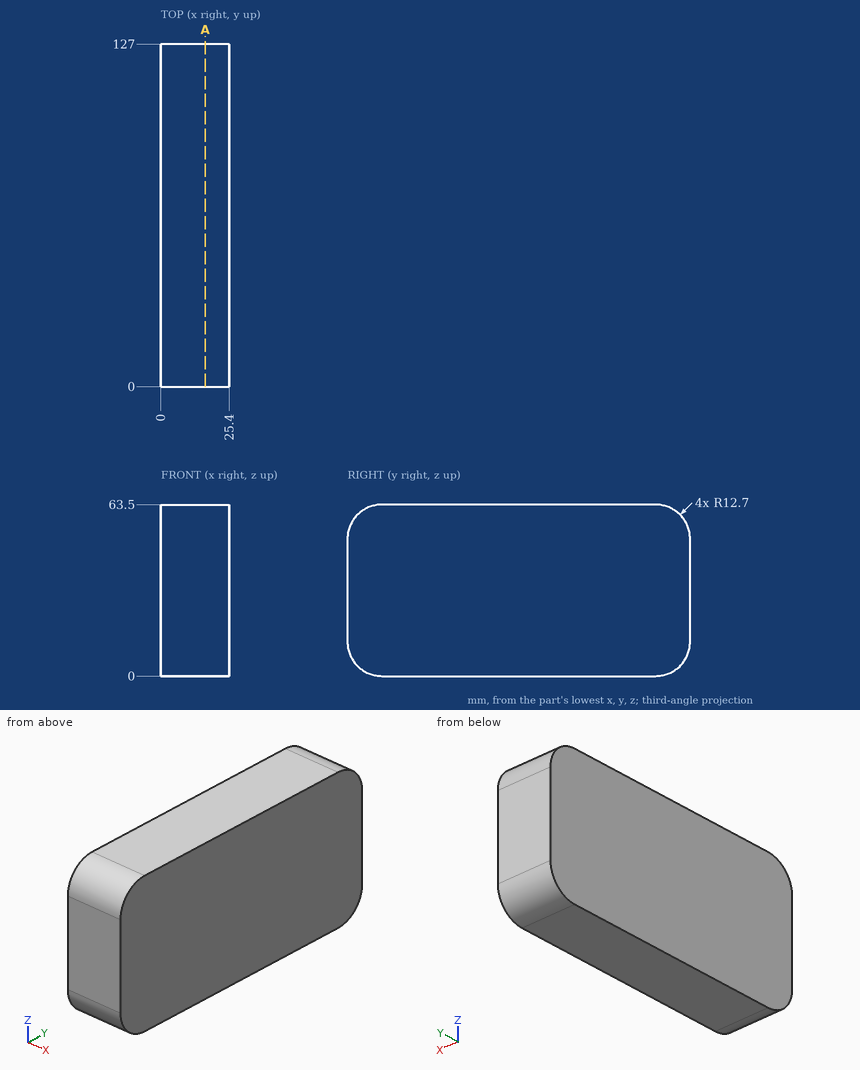
Design review of the part shown in the three views and the two pictorial views. Dimensions are in mm from the part's minimum x, y and z. Round coordinates to 2 decimals unless told otherwise and drop trailing zeros. Loops run counter-clockwise (first coordinate to the right, second up) from the corner with the lowest first, then second, coordinate; pieces in that order, holes last. Notation, with made-up numbers: (-2, -21.5) -> (49, -21.5) arc R15 ccw to (49, -12.5) -> close; hole circle Ø2 at (61.25, 25.5). An arc over 180 degrees is marked (long way). Use one line per item in the form item = value. Start each with the question number.
Q1. Wall thickness on line 1 along Z through (x, y) = (13.5, 114.5); line 2 along Y through (x, z) = (11.25, 55.5); line 3 along Z through (x, y) = (2.75, 117): over which ranges is each line inside the solid? List them lowest first. Write a range as [from, to].
Q2. We need section A-A on x = 16.5. Give the boundary of the cut face in (y, z).
Q3. For pin 1 Ø1.5 at (x, z) = (9, 8) entering from -Y, flat-tipped, find the tip position at first contact; note if it passes through.
Calculated:
q1.line_1 = [0, 63.5]
q1.line_2 = [0.9, 126.1]
q1.line_3 = [0.29, 63.21]
q2.outline = (0, 12.7) arc R12.7 ccw to (12.7, 0) -> (114.3, 0) arc R12.7 ccw to (127, 12.7) -> (127, 50.8) arc R12.7 ccw to (114.3, 63.5) -> (12.7, 63.5) arc R12.7 ccw to (0, 50.8) -> close
q3.pin_1 = 0.63
